Design review of the part built by this model. Coordinates are the model's own, in mm. A direction names the side the tool comes from. Give positions to 0.01 mm unless a question says otherwise; leave off trailing zeros. Loops run counter-clockwise (first coordinate to the right, second up) from the corner with the lowest first, then second, coordinate; pieces in that order, holes last. Notation, with made-up numbers: (-13, -28.75) - (30, -28.75) arc R22 ccw to (30, 7.25) - close; hole circle Ø8 at (80, 34.5). An arc over 180 degrees is marked (long way). One line per item, written item: value. Start each with the question number.
```python
from build123d import *

# Parameters (mm, degrees)
PAD012_DEPTH    = 10
SKETCH027_W     = 3.4
SKETCH027_H     = 5
POCKET_DEPTH    = 30
POCKET012_DEPTH = 63.499031
SKETCH029_R     = 11
POCKET013_DEPTH = 3.5
POCKET014_DEPTH = 5
SKETCH031_R     = 2.2
POCKET015_DEPTH = 5.001
POCKET016_DEPTH = 243.669334
FILLET_R        = 0.5
FILLET001_R     = 1
FILLET002_R     = 1


with BuildPart() as part:
    # Sketch026 (on ShapeBinder) → Pad012 (new body)
    with BuildSketch(Plane.XZ.offset(47.5)):
        with BuildLine():
            ThreePointArc((18, -27.658633), (33, 0), (18, 27.658633))
            Line((18, 27.658633), (9, 27.658633))
            Line((9, 31.749016), (9, 27.658633))
            Line((-9, 31.749016), (9, 31.749016))
            Line((-9, 31.749016), (-9, 27.658633))
            Line((-18, 27.658633), (-9, 27.658633))
            ThreePointArc((-18, 27.658633), (-33, 0), (-18, -27.658633))
            Line((-18, -27.658633), (-9, -27.658633))
            Line((-9, -31.749016), (-9, -27.658633))
            Line((-9, -31.749016), (9, -31.749016))
            Line((9, -31.749016), (9, -27.658633))
            Line((18, -27.658633), (9, -27.658633))
        make_face()
        with BuildLine():
            ThreePointArc((-1.45, -12.6), (0, -14.05), (1.45, -12.6))
            Line((1.45, -12.6), (1.45, -11.15))
            ThreePointArc((1.45, -11.15), (0, -9.7), (-1.45, -11.15))
            Line((-1.45, -12.6), (-1.45, -11.15))
        make_face(mode=Mode.SUBTRACT)
    extrude(amount=PAD012_DEPTH)

    # Sketch027 (on Face4 of Pad012) → Pocket (cut)
    with BuildSketch(Plane(origin=(0, -4.5, 31.749016), x_dir=(1, 0, 0), z_dir=(0, 0, 1))):
        with Locations((0, -45.5)):
            Rectangle(SKETCH027_W, SKETCH027_H)
    extrude(amount=-POCKET_DEPTH, mode=Mode.SUBTRACT)

    # Sketch028 (on Face14 of Pocket) → Pocket012 (cut, through all)
    with BuildSketch(Plane(origin=(0, -4.5, 31.749016), x_dir=(1, 0, 0), z_dir=(0, 0, 1))):
        with BuildLine():
            Line((-6.074874, -48.75), (-4.625126, -48.75))
            Line((-4.112563, -49.262563), (-4.625126, -48.75))
            ThreePointArc((-6.587437, -49.262563), (-5.35, -52.25), (-4.112563, -49.262563))
            Line((-6.074874, -48.75), (-6.587437, -49.262563))
        make_face()
        with BuildLine():
            Line((4.625126, -48.75), (6.074874, -48.75))
            Line((6.587437, -49.262563), (6.074874, -48.75))
            ThreePointArc((4.112563, -49.262563), (5.35, -52.25), (6.587437, -49.262563))
            Line((4.625126, -48.75), (4.112563, -49.262563))
        make_face()
    extrude(amount=-POCKET012_DEPTH, mode=Mode.SUBTRACT)

    # Sketch029 (on Face4 of Pocket012) → Pocket013 (cut)
    with BuildSketch(Plane(origin=(0, -47.5, 0), x_dir=(-1, 0, 0), z_dir=(0, 1, 0))):
        with Locations((0, -12.6)):
            Circle(SKETCH029_R)
    extrude(amount=-POCKET013_DEPTH, mode=Mode.SUBTRACT)

    # Sketch030 (on Face5 of Pocket013) → Pocket014 (cut)
    with BuildSketch(Plane.XZ.offset(57.5)):
        Polygon((27.036196, -16.3), (29.172392, -12.6), (27.036196, -8.9), (22.763804, -8.9), (20.627608, -12.6), (22.763804, -16.3), align=None)
        Polygon((-22.763804, -16.3), (-20.627608, -12.6), (-22.763804, -8.9), (-27.036196, -8.9), (-29.172392, -12.6), (-27.036196, -16.3), align=None)
    extrude(amount=-POCKET014_DEPTH, mode=Mode.SUBTRACT)

    # Sketch031 (on Face46 of Pocket014) → Pocket015 (cut, through all)
    with BuildSketch(Plane.XZ.offset(52.5)):
        with Locations((24.9, -12.6)):
            Circle(SKETCH031_R)
        with Locations((-24.9, -12.6)):
            Circle(SKETCH031_R)
    extrude(amount=-POCKET015_DEPTH, mode=Mode.SUBTRACT)

    # Sketch032 (on Face3 of Pocket015) → Pocket016 (cut, through all)
    with BuildSketch(Plane(origin=(0, -4.5, 27.658633), x_dir=(1, 0, 0), z_dir=(0, 0, 1))):
        with BuildLine():
            Line((11.025126, -48.75), (12.474874, -48.75))
            Line((12.474874, -48.75), (12.987437, -49.262563))
            ThreePointArc((10.512563, -49.262563), (11.75, -52.25), (12.987437, -49.262563))
            Line((11.025126, -48.75), (10.512563, -49.262563))
        make_face()
        with BuildLine():
            Line((15.025126, -44.125), (16.474874, -44.125))
            Line((16.474874, -44.125), (16.987437, -44.637563))
            ThreePointArc((14.512563, -44.637563), (15.75, -47.625), (16.987437, -44.637563))
            Line((15.025126, -44.125), (14.512563, -44.637563))
        make_face()
    pocket016 = extrude(amount=-POCKET016_DEPTH, mode=Mode.SUBTRACT)

    # Mirrored: Pocket016 across Sketch032 V_Axis
    add(pocket016.mirror(Plane(origin=(0, -4.5, 27.658633), x_dir=(0, 0, 1), z_dir=(1, 0, 0))), mode=Mode.SUBTRACT)

    # Fillet
    fillet_edges = [part.edges().sort_by_distance(p)[0] for p in [
        (-1.7, -52.5, 16.749016),
        (1.7, -52.5, 16.749016),
    ]]
    fillet(fillet_edges, radius=FILLET_R)

    # Fillet001
    fillet001_edges = [part.edges().sort_by_distance(p)[0] for p in [
        (-9, -52.5, 31.749016),
        (9, -52.5, 31.749016),
    ]]
    fillet(fillet001_edges, radius=FILLET001_R)

    # Fillet002
    fillet002_edges = [part.edges().sort_by_distance(p)[0] for p in [
        (9, -52.5, -31.749016),
        (-9, -52.5, -31.749016),
    ]]
    fillet(fillet002_edges, radius=FILLET002_R)


solid = part.part
```
(1) Take a section at C-C on x = -24.9. State the section outline as (y, z) points.
(2) Take a section at A-A on z = 5.5. State how many separate pieces and enclosed holes the cut face has, and give its area (3 significant figures).
(3) Draft analysis for pull direction X (two halves, no side actions). For faces 5 (the flat face through (-9, -52, 29)), 6 (the flat face through (-5, -53.25, 0)), 7 (the flat face through (16, -48.625, 0)), 8 (the flat face through (0, -57.5, 0)), state which applies: pulls with the +X half, pulls with the -X half, needs draft (parallel to the pull), parting line crosses it, or undercut.
(4) To check wall thickness, follow L1, parallel to X at y = -50, z = -1.5; L2, parallel to X at y = -51, z = 0; L3, parallel to Y at x = 11.5, z = 20.5. State the ranges of each line that lie inside material, in increasing order. Write a range as from..to.
(5) For pin 1 Ø4.5 at (x, y) = (25.5, -55) entering from -Z; pin 2 Ø3 at (y, z) = (-54.5, -13) entering from +X; pin 3 Ø6 at (y, z) = (-56.5, -19) entering from +X; pin 4 Ø6 at (x, y) = (-8.5, -56) entering from -Z, all flat-tipped, find the tip position at first contact; note any pin that passes through.
(6) Machinability: for faces 1 (the cylindrical face through (8.73, -49.23, -19.29)), 2 (the flat face through (1.45, -54, -12)), 3 (the flat face through (0, -50, 1.749)), 4 (the flat face through (27, -52.5, -11)), which of the approach directions +Z, -Z, +X, -X, +Y, -Y give a long, thin tool a straight path to every point of the face, cutting with its end or side? Answer none if there is none.
Here are the results:
1. outline: (-57.5, -21.66) - (-47.5, -21.66) - (-47.5, -14.8) - (-52.5, -14.8) - (-52.5, -16.3) - (-57.5, -16.3) - close; (-57.5, -8.9) - (-52.5, -8.9) - (-52.5, -10.4) - (-47.5, -10.4) - (-47.5, 21.66) - (-57.5, 21.66) - close
2. separate pieces: 1
2. enclosed holes: 6
2. area: 575 mm²
3. face 5: pulls with the -X half
3. face 6: undercut
3. face 7: undercut
3. face 8: needs draft
4. L1: -32.97..-17.46, -14.04..14.04, 17.46..32.97
4. L2: -33..-17.38, -14.12..14.12, 17.38..33
4. L3: -57.5..-56.73, -53.25..-47.5
5. pin 1: z = -23.42
5. pin 2: x = 30.93
5. pin 3: x = 28.86
5. pin 4: z = -31.75
6. face 1: +Y
6. face 2: +Y, -Y
6. face 3: +Z, +Y
6. face 4: -Y
